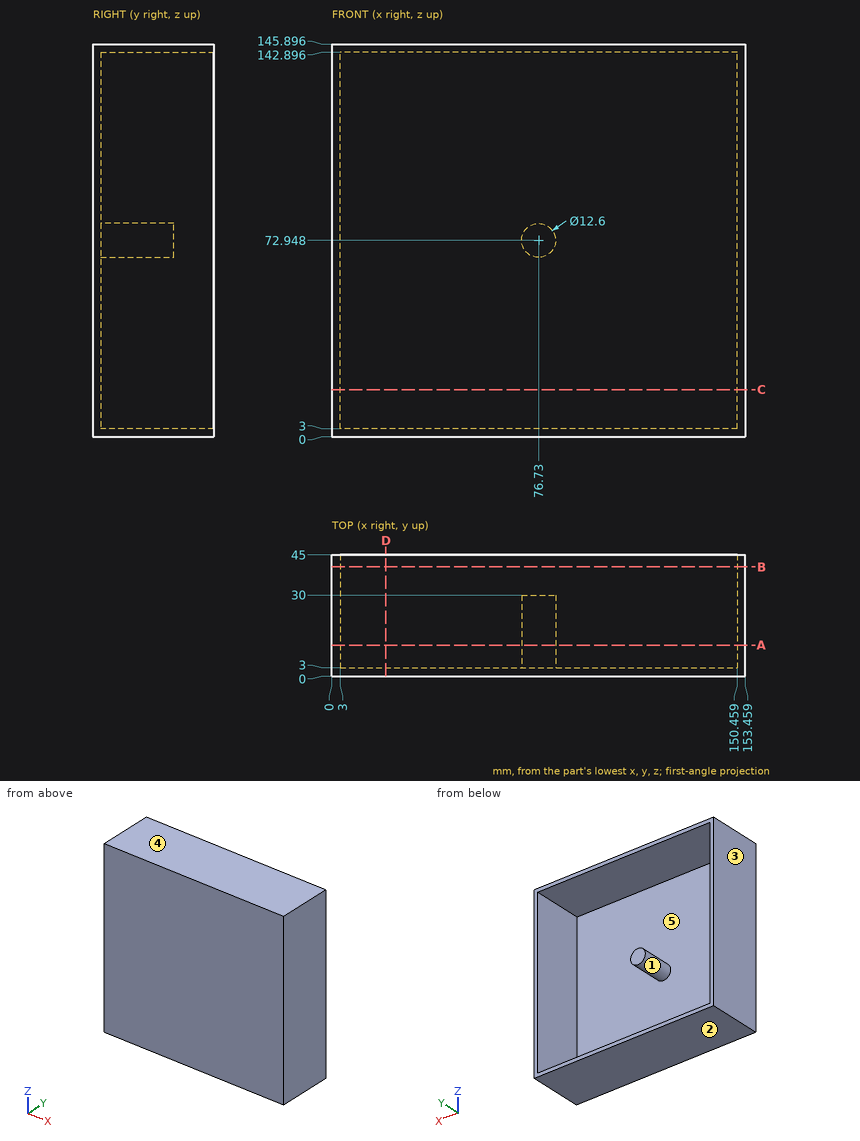
Input: dimensioned drawing with shaded views. Units: mm. Origin: part minimum x, y, z. A direction names the side the tool comes from. Round coordinates to 2 decimals unless told otherwise and drop trailing zeros. Loops run counter-clockwise (first coordinate to the right, second up) from the corner with the lowest first, then second, coordinate; pieces in that order, holes last. Notation, with made-up numbers: (-21.75, 31) -> (34.25, 31) arc R19 ccw to (34.25, 55) -> close; hole circle Ø11 at (-4.75, 81.5). An arc over 180 degrees is marked (long way). One line per item, written item: value.
(1) Section C-C (z = 17.5). Return the cut outline in (x, y).
Geometry check:
outline: (0, 0) -> (153.46, 0) -> (153.46, 45) -> (150.46, 45) -> (150.46, 3) -> (3, 3) -> (3, 45) -> (0, 45) -> close
(2) Set-up query: the marked faces 4 and 5. Return all of +Z, -Z, +X, -X, +Y, -Y with unobstructed straight access to the full face (end or side cutting, diameter ignored); none if empty.
Geometry check:
face 4: +Z, +X, -X, +Y, -Y
face 5: +Y
(3) Material intervals for line 1 (X direction, y = 40.5, z = 68.5); line 2 (Z direction, x = 77, y = 23.5) (1 decimal); line 3 (Z direction, x = 47, y = 28.5) (1 decimal), sorted ascending. Write a range as [from, to].
Geometry check:
line 1: [0, 3], [150.46, 153.46]
line 2: [0, 3], [66.7, 79.2], [142.9, 145.9]
line 3: [0, 3], [142.9, 145.9]
(4) Section B-B (y = 40.5). Return the cut outline in (x, z) (1 decimal), plus the area to 3 significant figures.
Geometry check:
outline: (0, 0) -> (153.5, 0) -> (153.5, 145.9) -> (0, 145.9) -> close; hole (3, 3) -> (150.5, 3) -> (150.5, 142.9) -> (3, 142.9) -> close
area: 1,760 mm2
(5) Section A-A (y = 11.5). Return the cut outline in (x, z) (1 decimal).
Geometry check:
outline: (0, 0) -> (153.5, 0) -> (153.5, 145.9) -> (0, 145.9) -> close; circle Ø12.6 at (76.7, 72.9); hole (3, 3) -> (150.5, 3) -> (150.5, 142.9) -> (3, 142.9) -> close
(6) Pin query (flat end, axial travel): pin 1 (21 mm diameter, centred on y = 14.5, z = 96.5, fed in from -X); pin 2 (5 mm diameter, centred on x = 57.5, z = 54.5, fed in from +Y); pin 3 (14 mm diameter, centred on x = 75, z = 72.5, fed in from +Y). Return the tip coordinate at first contact, or that it passes through.
Geometry check:
pin 1: x = 0
pin 2: y = 3
pin 3: y = 30
(7) Mould query, pull axis X, two halves, no side actions, for the marked faces 1, 2 and 3. Classes: pulls with the +X half, pulls with the -X half, needs draft (parallel to the pull), parting line crosses it, or undercut.
Geometry check:
face 1: undercut
face 2: needs draft
face 3: pulls with the -X half
(8) Section D-D (x = 20). Return the cut outline in (y, z) (1 decimal).
Geometry check:
outline: (0, 0) -> (45, 0) -> (45, 3) -> (3, 3) -> (3, 142.9) -> (45, 142.9) -> (45, 145.9) -> (0, 145.9) -> close
